Geometry check sheet. Reference: the model listing, model coordinates, mm. Give positions to 0.01 mm unless a question says otherwise; leave off trailing zeros. Order: outer loops, then holes, each group sorted by start corner. A loop starts at its lowest first (then second) coordinate and runs counter-clockwise, first axis right, second up. Notation, with made-up numbers: (-26, 75) - (7, 75) arc R11 cw to (7, 85) - close; hole circle Ø3 at (50, 4). An arc over 180 degrees is marked (long way). Put each result on its own line as item: value. Start each with the question number.
```python
from build123d import *

# Parameters (mm, degrees)
SKETCH1_W           = 28
SKETCH1_H           = 15
BOSS_EXTRUDE1_DEPTH = 4
SKETCH3_R           = 4
SKETCH3_R_2         = 1.65
BOSS_EXTRUDE2_DEPTH = 4
SKETCH5_W           = 12
SKETCH5_H           = 15
SKETCH5_R           = 1.6
BOSS_EXTRUDE3_DEPTH = 4
FILLET1_R           = 3
CUT_EXTRUDE1_DEPTH  = 15


with BuildPart() as part:
    # Sketch1 → Boss-Extrude1 (new body)
    with BuildSketch(Plane.XY):
        Rectangle(SKETCH1_W, SKETCH1_H)
    extrude(amount=BOSS_EXTRUDE1_DEPTH)

    # Sketch3 → Boss-Extrude2 (add)
    with BuildSketch(Plane.ZY.offset(14)):
        with BuildLine():
            Line((10.609415807, 3.397699996), (4, 7.5))
            Line((4, 7.5), (4, -7.5))
            Line((4, -7.5), (10.608760269, -3.399872364))
            ThreePointArc((10.608760269, -3.399872364), (4.500000019, -0.000497042), (10.609415807, 3.397699996))
        make_face()
        with Locations((8.5, -0.00088279)):
            Circle(SKETCH3_R)
        with Locations((8.5, -0.00088279)):
            Circle(SKETCH3_R_2, mode=Mode.SUBTRACT)
    boss_extrude2 = extrude(amount=-BOSS_EXTRUDE2_DEPTH)

    # Sketch5 → Boss-Extrude3 (add)
    with BuildSketch(Plane(origin=(0, 0, 0), x_dir=(-1, 0, 0), z_dir=(0, 0, -1))):
        with Locations((20, 0)):
            Rectangle(SKETCH5_W, SKETCH5_H)
        with Locations((20, 0)):
            Circle(SKETCH5_R, mode=Mode.SUBTRACT)
    boss_extrude3 = extrude(amount=-BOSS_EXTRUDE3_DEPTH)

    # Mirror1: Boss-Extrude2, Boss-Extrude3 across plane
    add(boss_extrude2.mirror(Plane(origin=(0, 0, 0), x_dir=(0, 0, 1), z_dir=(1, 0, 0))))
    add(boss_extrude3.mirror(Plane(origin=(0, 0, 0), x_dir=(0, 0, 1), z_dir=(1, 0, 0))))

    # Fillet1
    fillet1_edges = [part.edges().sort_by_distance(p)[0] for p in [
        (-26, 7.5, 2),
        (-26, -7.5, 2),
        (26, 7.5, 2),
        (26, -7.5, 2),
    ]]
    fillet(fillet1_edges, radius=FILLET1_R)

    # Sketch6 → Cut-Extrude1 (cut)
    with BuildSketch(Plane.XZ.offset(7.5)):
        Polygon((0, 0), (37.280314588, 0), (37.280314588, 22.501925167), (0, 22.501925167), (-10, 22.501925167), (-10, 0), align=None)
    extrude(amount=-CUT_EXTRUDE1_DEPTH, mode=Mode.SUBTRACT)


solid = part.part
```
Item 1: Cross-section at C-C (z = 8.5). Enter the section's corners in (x, y), and give its area (3 significant figures).
Item 2: Thickness scan on line 1 along Y through (x, z) = (-20, 2.85); line 2 along X through (y, z) = (-5.75, 5.75); line 3 along Z through (x, y) = (-16, 0.25). Record the ranges inside material, lowest first.
Item 3: Cross-section at D-D (y = 0.5). Enter the section's corners in (x, z).
Item 4: Release check for a two-part mould opening along X. For faces 1 (the face through (-18.82, 1.08, 1.97)), 2 (the face through (-20, 2, 4)), 3 (the face through (-14, 0, 6)), 4 (the face through (-10, 0, 5)) record: +X half, -X half, draft (parallel to the pull), parting line (faces both ways), or undercut.
Item 5: Gauge pin test, flat ends, axial feed: pin 1 Ø3 at (y, z) = (0, 8.5) entering from +X; pin 2 Ø4 at (x, y) = (-18, 3) entering from +Z; pin 3 Ø2.5 at (y, z) = (-3, 9) entering from -X; pin 4 Ø3 at (x, z) = (-15, 7) entering from +Y. Record the tip position at first contact, or that the pin passes through.
Item 6: Cross-section at B-B (x = -20). Enter the section's corners in (y, z), and give its area (3 significant figures).
Item 7: Cross-section at A-A (z = 2.75). Enter the section's corners in (x, y), and give its area (3 significant figures).
Recorded:
1. outline: (-14, -4.71) - (-10, -4.71) - (-10, -1.65) - (-14, -1.65) - close; (-14, 1.65) - (-10, 1.65) - (-10, 4.71) - (-14, 4.71) - close
1. area: 24.5 mm^2
2. line 1: y = -7.5 to -1.6, 1.6 to 7.5
2. line 2: x = -14 to -10
2. line 3: z = 0 to 4
3. outline: (-26, 0) - (-21.52, 0) - (-21.52, 4) - (-26, 4) - close; (-18.48, 0) - (-10, 0) - (-10, 6.93) - (-14, 6.93) - (-14, 4) - (-18.48, 4) - close; (-14, 10.07) - (-10, 10.07) - (-10, 12.47) - (-14, 12.47) - close
4. face 1: undercut
4. face 2: draft
4. face 3: -X half
4. face 4: +X half
5. pin 1: passes through
5. pin 2: stops at z = 4
5. pin 3: stops at x = -14
5. pin 4: stops at y = 6.33
6. outline: (-7.5, 0) - (-1.6, 0) - (-1.6, 4) - (-7.5, 4) - close; (1.6, 0) - (7.5, 0) - (7.5, 4) - (1.6, 4) - close
6. area: 47.2 mm^2
7. outline: (-26, -4.5) arc R3 ccw to (-23, -7.5) - (-10, -7.5) - (-10, 7.5) - (-23, 7.5) arc R3 ccw to (-26, 4.5) - close; hole circle Ø3.2 at (-20, 0)
7. area: 228 mm^2
